Here's how the part is built. I have some questions about the finished solid (model axes, mm). A direction names the side the tool comes from. Round coordinates to 2 decimals unless told otherwise and drop trailing zeros. Order: outer loops, then holes, each group sorted by start corner. A loop starts at its lowest first (then second) coordinate and runs counter-clockwise, first axis right, second up. Notation, with made-up numbers: (42, -4.75) -> (46, -4.75) arc R7 ccw to (46, 3.25) -> close; hole circle Ø1 at (-4, 65). An arc over 180 degrees is marked (long way). Use a Markdown table: item, result. Add a question column.
from build123d import *

# Parameters (mm, degrees)
BOSS_EXTRUDE1_DEPTH = 190.5
SKETCH2_R           = 127
BOSS_EXTRUDE2_DEPTH = 101.6
SKETCH3_R           = 74.295
BOSS_EXTRUDE3_DEPTH = 46.228
SKETCH4_R           = 74.295
BOSS_EXTRUDE4_DEPTH = 46.228
SKETCH6_W           = 25.4
SKETCH6_H           = 50.8
BOSS_EXTRUDE5_DEPTH = 25.4
SKETCH7_R           = 12.7
CUT_EXTRUDE1_DEPTH  = 73.152


with BuildPart() as part:
    # Sketch1 → Boss-Extrude1 (new body)
    with BuildSketch(Plane(origin=(0, 0, 0), x_dir=(1, 0, 0), z_dir=(0, 1, 0))):
        Polygon((260.35, 508), (260.35, 431.8), (714.502, 431.8), (714.502, 76.2), (260.35, 76.2), (260.35, 0), (0, 0), (0, 508), align=None)
    extrude(amount=BOSS_EXTRUDE1_DEPTH)

    # Sketch2 → Boss-Extrude2 (add)
    with BuildSketch(Plane.XY):
        with Locations(Location((260.35, 95.25, 0), (0, 0, 228.590377891))):
            Circle(SKETCH2_R)
    boss_extrude2 = extrude(amount=BOSS_EXTRUDE2_DEPTH)

    # Sketch3 → Boss-Extrude3 (add)
    with BuildSketch(Plane.XY):
        with Locations(Location((0, 42.418, 0), (0, 0, 90))):
            Circle(SKETCH3_R)
    boss_extrude3 = extrude(amount=BOSS_EXTRUDE3_DEPTH)

    # Sketch4 → Boss-Extrude4 (add)
    with BuildSketch(Plane.XY.offset(-76.2)):
        with Locations(Location((714.502, 42.418, 0), (0, 0, 214.815812785))):
            Circle(SKETCH4_R)
    boss_extrude4 = extrude(amount=BOSS_EXTRUDE4_DEPTH)

    # Mirror1: Boss-Extrude2, Boss-Extrude3, Boss-Extrude4 across plane
    add(boss_extrude2.mirror(Plane.XY.offset(-254)))
    add(boss_extrude3.mirror(Plane.XY.offset(-254)))
    add(boss_extrude4.mirror(Plane.XY.offset(-254)))

    # Sketch6 → Boss-Extrude5 (add, symmetric)
    with BuildSketch(Plane.ZY.offset(-330.2)):
        with Locations((-88.9, 215.9)):
            Rectangle(SKETCH6_W, SKETCH6_H)
    boss_extrude5 = extrude(amount=BOSS_EXTRUDE5_DEPTH, both=True)

    # Sketch7 → Cut-Extrude1 (cut)
    with BuildSketch(Plane(origin=(0, 0, -101.6), x_dir=(-1, 0, 0), z_dir=(0, 0, -1))):
        with Locations((-330.2, 215.9)):
            Circle(SKETCH7_R)
    cut_extrude1 = extrude(amount=-CUT_EXTRUDE1_DEPTH, mode=Mode.SUBTRACT)

    # Mirror2: Boss-Extrude5, Cut-Extrude1 across plane
    add(boss_extrude5.mirror(Plane.XY.offset(-254)))
    add(cut_extrude1.mirror(Plane.XY.offset(-254)), mode=Mode.SUBTRACT)


solid = part.part
(1) I'm going to push flat-ended pins straight in: P1, Ø6, axis at y = 1.5, z = -71.5, coming from the +X side; P2, Ø8, axis at x = 300.5, z = -388, coming from the -Y side; P3, Ø2, axis at x = 641, z = -267, coming from the +Y side. Where does each tip first touch, or does it pass through?
(2) I want a section at D-D on z = -193.5. List the corners of the cut face in (x, y) for me.
(3) I want a section at A-A on x = 330.2. List the corners of the cut face in (y, z) for me, and give its area (3 significant figures).
(4) On a 3-axis mill with a long thin cutter (end or side, diameter ignored), from which of +Z, -Z, +X, -X, +Y, -Y can I reach the whole of each face in a straight line? I mean faces 1 (the flat face through (-1, 41, 46.228)), 2 (the flat face through (355.6, 216, -419)), 3 (the flat face through (716, 42, -478.028)). Say none if no direction works.
(5) I want a section at B-B on x = 18. List the corners of the cut face in (y, z) for me, and give its area (3 significant figures).
(6) If we mould it in two halves opening along X, with no side actions, what happens to faces 4 (the flat face through (87, 115, -508)), 5 (the flat face through (-23, 41, -508)), 6 (the flat face through (304.8, 216, -419))? For each: pulls with the +X half, pulls with the -X half, needs draft (parallel to the pull), parting line crosses it, or undercut.
(7) Please list where these lines run through material, in increasing order: probe 1 along Z at (x, y) = (323.5, 22.5); probe 2 along X at (y, z) = (215, -413); probe 3 along Y at (x, z) = (330.2, -415.75). Write a range as from..to.
Output:
| question | item | result |
|---|---|---|
| 1 | P1 | x = 778.39 |
| 1 | P2 | y = 0 |
| 1 | P3 | y = 190.5 |
| 2 | outline | (0, 0) -> (714.5, 0) -> (714.5, 190.5) -> (0, 190.5) -> close |
| 3 | outline | (-10.82, -609.6) -> (201.32, -609.6) -> (201.32, -508) -> (-10.82, -508) -> close; (-10.82, 0) -> (201.32, 0) -> (201.32, 101.6) -> (-10.82, 101.6) -> close; (0, -431.8) -> (203.2, -431.8) -> (203.2, -406.4) -> (190.5, -406.4) -> (190.5, -101.6) -> (203.2, -101.6) -> (203.2, -76.2) -> (0, -76.2) -> close; (228.6, -431.8) -> (241.3, -431.8) -> (241.3, -406.4) -> (228.6, -406.4) -> close; (228.6, -101.6) -> (241.3, -101.6) -> (241.3, -76.2) -> (228.6, -76.2) -> close |
| 3 | area | 112,000 mm² |
| 4 | face 1 | +Z, -X, +Y, -Y |
| 4 | face 2 | +Z, -Z, +X, +Y |
| 4 | face 3 | -Z, +X, +Y, -Y |
| 5 | outline | (-29.66, -554.23) -> (114.5, -554.23) -> (114.5, -508) -> (190.5, -508) -> (190.5, 0) -> (114.5, 0) -> (114.5, 46.23) -> (-29.66, 46.23) -> (-29.66, 0) -> (0, 0) -> (0, -508) -> (-29.66, -508) -> close |
| 5 | area | 110,000 mm² |
| 6 | face 4 | undercut |
| 6 | face 5 | needs draft |
| 6 | face 6 | pulls with the -X half |
| 7 | probe 1 | -609.6..-508, -431.8..-76.2, 0..101.6 |
| 7 | probe 2 | 304.8..317.53, 342.87..355.6 |
| 7 | probe 3 | 0..203.2, 228.6..241.3 |
